Print and shaded views of the part. All mm, measured from the part's lowest x, y and z. A direction names the side the tool comes from. Coordinates: 2 decimals unless noted, no trailing zeros. Loops run counter-clockwise (first coordinate to the right, second up) from the corner with the lowest first, then second, coordinate; pieces in that order, holes last. Notation, with made-up numbers: (24, 42) -> (83, 42) arc R20 ccw to (83, 79) -> close; hole circle Ø7 at (22, 19). An arc over 180 degrees is marked (long way). One line per question, with ' | ' between items. Start each with the question number.
1) Probe L1, parallel to Z at x = 14, y = 9; L2, parallel to X at y = 9.75, z = 6.5; L3, parallel to X at y = 6.5, z = 1.75. List the from-to ranges inside material, lowest first. Write a range as from..to.
2) Cut at A-A (x = 26.67). List the corners of the cut face in (y, z) (1 decimal).
3) Cut at B-B (z = 6.5). List the corners of the cut face in (x, y).
4) 3-axis set-ups, long thin cutter, end or side, ignore diameter. For the marked faces 1, 2 and 3: which of +Z, -Z, +X, -X, +Y, -Y reach the whole face in a straight line?
5) Drop a flat-ended pin along its axis: pin 1 (4 mm diameter, centred on x = 17, y = 3.5, fed in from -Z). Give the stop position or say it passes through.
6) Cut at C-C (y = 8). List the corners of the cut face in (x, z), plus the area to 3 significant figures.
7) Cut at D-D (x = 16). List the corners of the cut face in (y, z).
8) Two-plate mould, pull along X, no slides. Class the marked faces 4, 5 and 6: released by +X, released by -X, zero draft, split by the parting line, or undercut.
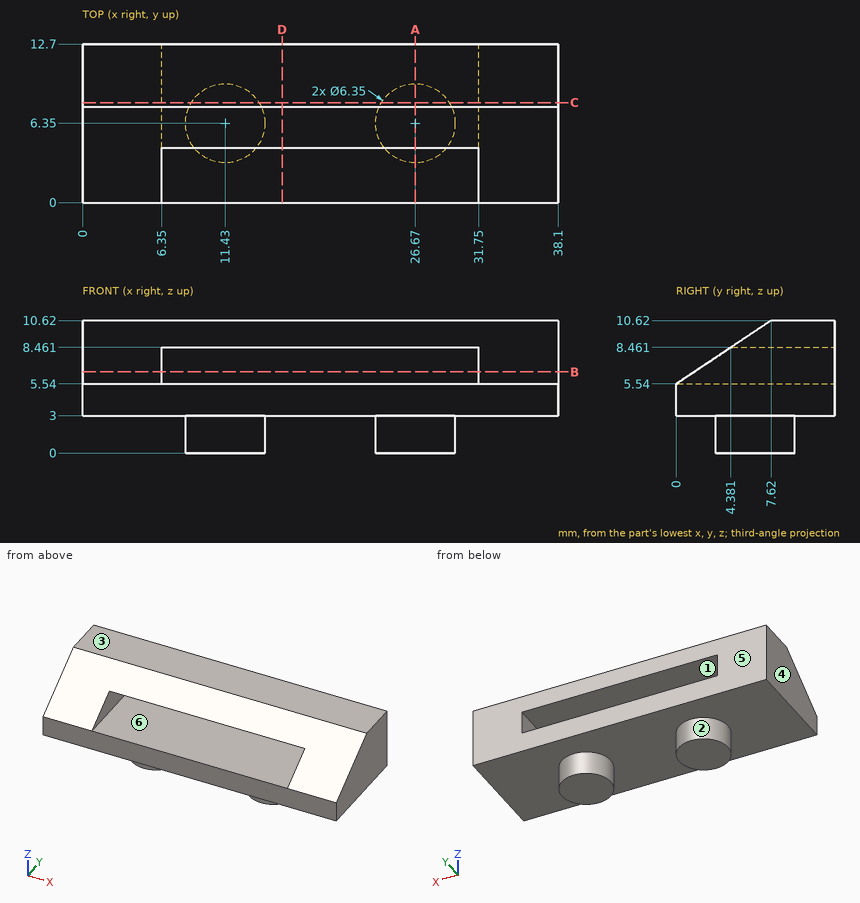
Reported:
1) L1: z = 3..5.54, 8.46..10.62 | L2: x = 0..6.35, 31.75..38.1 | L3: x = 8.26..14.6, 23.5..29.84
2) outline: (0, 3) -> (3.2, 3) -> (3.2, 0) -> (9.5, 0) -> (9.5, 3) -> (12.7, 3) -> (12.7, 5.5) -> (0, 5.5) -> close; (4.4, 8.5) -> (12.7, 8.5) -> (12.7, 10.6) -> (7.6, 10.6) -> close
3) outline: (0, 1.44) -> (6.35, 1.44) -> (6.35, 12.7) -> (0, 12.7) -> close; (31.75, 1.44) -> (38.1, 1.44) -> (38.1, 12.7) -> (31.75, 12.7) -> close
4) face 1: +Y, -Y | face 2: -Z | face 3: +Z, +X, -X, +Y, -Y
5) pin 1: stops at z = 3
6) outline: (0, 3) -> (8.72, 3) -> (8.72, 0) -> (14.14, 0) -> (14.14, 3) -> (23.96, 3) -> (23.96, 0) -> (29.38, 0) -> (29.38, 3) -> (38.1, 3) -> (38.1, 10.62) -> (0, 10.62) -> close; hole (6.35, 5.54) -> (31.75, 5.54) -> (31.75, 8.46) -> (6.35, 8.46) -> close | area: 249 mm²
7) outline: (0, 3) -> (12.7, 3) -> (12.7, 5.54) -> (0, 5.54) -> close; (4.38, 8.46) -> (12.7, 8.46) -> (12.7, 10.62) -> (7.62, 10.62) -> close
8) face 4: released by -X | face 5: zero draft | face 6: undercut
